Design review of the part built by this model. Coordinates are the model's own, in mm. A direction names the side the tool comes from. Coordinates: 2 decimals unless noted, no trailing zeros. Loops run counter-clockwise (first coordinate to the right, second up) from the corner with the lowest first, then second, coordinate; pieces in that order, holes last.
Q1. Machinability: for faces 1 (the face through (-59.473, 7.937, 136.998)), 2 (the face through (-27.02, 53.57, 118.54)), 3 (the face through (0, 37, 15)), 4 (the face through (-24, -23, 100)), which of the approach directions +Z, -Z, +X, -X, +Y, -Y give a long, thin tool a straight path to every point of the face, cutting with its end or side? Answer none if there is none.
Q2. For P1, Ø10, axis at x = -35.5, y = 67, coming from the +Z side; P2, Ø18, axis at x = -23, y = -13, coming from the +Z side; P3, Ø18, axis at x = -28.5, y = -15.5, coming from the -Z side, all flat-tipped, find the tip position at first contact; note any pin that passes through.
Q3. Add section A-A on y = -48. Give the boundary of the cut face in (x, z).
Q4. Wall thickness on probe 1 along Y at (x, z) = (-105.5, 65); probe 2 along X at (y, z) = (38.5, 109); probe 3 along Z at (x, y) = (-107.5, 16.5): over which ranges is each line inside the solid? List them lowest first.
Autodesk Inventor part; units mm, degrees
ref_plane "YZ Plane" through (0, 0, 0) normal (1, 0, 0) x (0, 1, 0)
ref_plane "XZ Plane" through (0, 0, 0) normal (0, 1, 0) x (-1, 0, 0)
sketch "Esquisse1" plane through (0, 0, 0) normal (0, 0, 1) x (1, 0, 0)
  line L0 (0, 0) -> (160, 0) construction
  line L1 (0, 0) -> (0, 100) construction
  line L2 (0, 100) -> (87.1369, 86.9657) construction
  line L3 (87.1369, 86.9657) -> (160, 0) construction
  spline S0 degree 2 poles (0, 100) (87.1369, 86.9657) (160, 0) knots 1 1 1 2 2 2
  line L4 (0, 100) -> (0, 0)
  line L5 (0, 0) -> (160, 0)
  dimension "d0" = 160
  dimension "d1" = 100
revolve "Révolution1" add sketch "Esquisse1" angle 360 about axis through (0, 0, 0) along (0, 1, 0)
ref_plane "Plan de construction1" through (0, 0, 130) normal (0, 0, 1) x (1, 0, 0)
sketch "Esquisse3" plane through (0, 0, 130) normal (0, 0, 1) x (1, 0, 0)
  circle A0 centre (0, 0) radius 60
  dimension "d8" = 120
extrude "Extrusion2" add sketch "Esquisse3" against normal blind 30
sketch "Esquisse4" plane through (0, 0, 130) normal (0, 0, 1) x (1, 0, 0)
  circle A0 centre (0, 0) radius 60
  dimension "d11" = 120
extrude "Extrusion3" cut sketch "Esquisse4" along normal blind 30
sketch "Esquisse6" plane through (0, 0, 130) normal (0, 0, 1) x (1, 0, 0)
  line L0 (0, 105.5344) -> (175.5316, 105.5344)
  line L1 (175.5316, 105.5344) -> (175.5316, -202.4537)
  line L2 (175.5316, -202.4537) -> (0, -202.4537)
  line L3 (0, -202.4537) -> (0, 105.5344)
  point P0 (0, 0)
extrude "Extrusion5" cut sketch "Esquisse6" along normal mid plane 800
properties part number "RightSide"
Entries:
1. face 1: +Z, +X, -Y
1. face 2: +Z, -X, +Y
1. face 3: +Z, -Z, +X, +Y, -Y
1. face 4: -Z, +X, -X, -Y
2. P1: stops at z = 86.68
2. P2: stops at z = 130
2. P3: stops at z = 100
3. outline: (-36, 100) - (0, 100) - (0, 130) - (-36, 130) - close
4. probe 1: y = 0 to 37.75
4. probe 2: x = -57.16 to 0
4. probe 3: z = -97.94 to 97.94
